Build history of the part. All positions in model axes, mm. A direction names the side the tool comes from. Coordinates: 2 decimals unless noted, no trailing zeros. Loops run counter-clockwise (first coordinate to the right, second up) from the corner with the lowest first, then second, coordinate; pieces in that order, holes last.
Item 1: Cut at A-A (x = 139). List the corners of the cut face in (y, z), and give its area (3 significant figures).
Item 2: Flat gauge pins, fed straight in: pin 1 (5 mm diameter, centred on x = 116.5, y = 33.5, fed in from -Z); pin 2 (5 mm diameter, centred on x = 128, z = 7.5, fed in from -Y); pin 3 (5 mm diameter, centred on y = 44, z = 9, fed in from +X). Where does each tip first touch, or does it go through?
Item 3: Mould opens along Y. For faces 3 (the face through (98, 43, 2.5)), 4 (the face through (21, 67.521, 7)), 5 (the face through (76.29, 45.39, 1.27)), 6 (the face through (98, 57.521, 7)) say: released by +Y, released by -Y, zero draft, split by the parting line, or undercut.
Item 4: Drill centre lines: line 1 along Z through (x, y) = (73.5, 36.5); line 2 along X through (y, z) = (35, 12); line 3 along Y through (x, z) = (102, 5.5). Where is each one in solid material? Low to high.
Item 5: Cut at C-C (y = 31.5). List the corners of the cut face in (x, z), and give its area (3 significant figures).
Item 6: Cut at B-B (z = 5.75). List the corners of the cut face in (x, y).
Item 7: 3-axis set-ups, long thin cutter, end or side, ignore diameter. For faces 1 (the face through (39.069, 42, 7)), 2 (the face through (156.06, 30.37, 13.77)): which of +Z, -Z, +X, -X, +Y, -Y reach the whole face in a straight line?
from build123d import *

# Parameters (mm, degrees)
F1_DEPTH = 15
F0_W     = 120
F0_H     = 30
F2_DEPTH = 2.5
F3_W     = 120
F3_H     = 2.5
F4_DEPTH = 30
F5_R     = 10
F6_R     = 3.5
F7_DEPTH = 25


with BuildPart() as f1:
    # F0 (on Top) → F1 (new body)
    with BuildSketch(Plane.XY):
        Polygon((159.068721, 67.520804), (-120.931279, 67.520804), (-120.931279, 27.520804), (39.068721, 27.520804), (39.068721, 57.520804), (159.068721, 57.520804), align=None)
    extrude(amount=F1_DEPTH)

    # F0 (on Top) → F2 (join)
    with BuildSketch(Plane.XY):
        with Locations((99.068721, 42.520804)):
            Rectangle(F0_W, F0_H)
    extrude(amount=F2_DEPTH)

    # F3 (on face) → F4 (join)
    with BuildSketch(Plane.XZ.offset(-57.520804)):
        with Locations((99.068721, 13.75)):
            Rectangle(F3_W, F3_H)
    extrude(amount=F4_DEPTH)

    # F5
    f5_edges = [f1.edges().sort_by_distance(p)[0] for p in [
        (159.068721, 27.520804, 13.75),
        (159.068721, 27.520804, 1.25),
    ]]
    fillet(f5_edges, radius=F5_R)

    # F6 (on face) → F7 (cut)
    with BuildSketch(Plane.XY.offset(15)):
        with Locations((79.068721, 47.520804)):
            Circle(F6_R)
        with Locations((119.068721, 47.520804)):
            Circle(F6_R)
    extrude(amount=-F7_DEPTH, mode=Mode.SUBTRACT)


solid = f1.part
Filled sheet:
1. outline: (27.52, 0) - (67.52, 0) - (67.52, 15) - (27.52, 15) - (27.52, 12.5) - (57.52, 12.5) - (57.52, 2.5) - (27.52, 2.5) - close
1. area: 300 mm2
2. pin 1: stops at z = 0
2. pin 2: stops at y = 57.52
2. pin 3: stops at x = 39.07
3. face 3: zero draft
3. face 4: released by +Y
3. face 5: undercut
3. face 6: released by -Y
4. line 1: z = 0 to 2.5, 12.5 to 15
4. line 2: x = -120.93 to 39.07
4. line 3: y = 57.52 to 67.52
5. outline: (-120.93, 0) - (157.05, 0) - (157.05, 2.5) - (39.07, 2.5) - (39.07, 12.5) - (157.05, 12.5) - (157.05, 15) - (-120.93, 15) - close
5. area: 2,990 mm2
6. outline: (-120.93, 27.52) - (39.07, 27.52) - (39.07, 57.52) - (159.07, 57.52) - (159.07, 67.52) - (-120.93, 67.52) - close
7. face 1: +X, -Y
7. face 2: +Z, -Z, +X, -Y
